CAD build for the part. Positions are in the model's coordinates, mm. Face numbers are marked on the shaded views. Give positions to 0.01 mm unless a question says otherwise; leave off trailing zeros. Loops run counter-clockwise (first coordinate to the right, second up) from the corner with the lowest first, then second, coordinate; pieces in that order, holes last. Notation, with made-up numbers: M 48.5,61 L 79.5,61 A28 ccw 79.5,87 Z; hole C 16.25,48 d11. An arc over 180 degrees is marked long. Answer as CSV lines item,"result".
```python
from build123d import *

# Parameters (mm, degrees)
EXTRUDE_1_DEPTH     = 2.5
FILLET_1_R          = 5
FILLET_2_R          = 5
FILLET_3_R          = 5
FILLET_4_R          = 5
SKETCH_2_R          = 3.5
SKETCH_2_R_2        = 1.54
SKETCH_2_R_3        = 5
CUT_EXTRUDE_2_DEPTH = 2.5
FILLET_5_R          = 3
FILLET_6_R          = 3
FILLET_7_R          = 3
FILLET_8_R          = 3
FILLET_9_R          = 3
FILLET_10_R         = 3
FILLET_11_R         = 3
FILLET_12_R         = 3


with BuildPart() as part:
    # 草图1 → 凸台-拉伸1 (new body)
    with BuildSketch(Plane.XY):
        Polygon((0, 13.5), (13.5, 0), (0, -13.5), (-13.5, 0), align=None)
    extrude(amount=EXTRUDE_1_DEPTH)

    # 圆角1
    fillet_1_edges = [part.edges().sort_by_distance(p)[0] for p in [
        (13.5, 0, 1.25),
    ]]
    fillet(fillet_1_edges, radius=FILLET_1_R)

    # 圆角2
    fillet_2_edges = [part.edges().sort_by_distance(p)[0] for p in [
        (0, -13.5, 1.25),
    ]]
    fillet(fillet_2_edges, radius=FILLET_2_R)

    # 圆角3
    fillet_3_edges = [part.edges().sort_by_distance(p)[0] for p in [
        (-13.5, 0, 1.25),
    ]]
    fillet(fillet_3_edges, radius=FILLET_3_R)

    # 圆角4
    fillet_4_edges = [part.edges().sort_by_distance(p)[0] for p in [
        (0, 13.5, 1.25),
    ]]
    fillet(fillet_4_edges, radius=FILLET_4_R)

    # 草图2 → 切除-拉伸2 (cut)
    with BuildSketch(Plane(origin=(0, 0, 0), x_dir=(-1, 0, 0), z_dir=(0, 0, -1))):
        Circle(SKETCH_2_R)
        with Locations((0, -6)):
            Circle(SKETCH_2_R_2)
        with Locations((0, 6)):
            Circle(SKETCH_2_R_2)
        with Locations((8, 0)):
            Circle(SKETCH_2_R_2)
        with Locations((-8, 0)):
            Circle(SKETCH_2_R_2)
        with Locations((8, 8)):
            Circle(SKETCH_2_R_3)
        with Locations((8, -8)):
            Circle(SKETCH_2_R_3)
        with Locations((-8, -8)):
            Circle(SKETCH_2_R_3)
        with Locations((-8, 8)):
            Circle(SKETCH_2_R_3)
    extrude(amount=-CUT_EXTRUDE_2_DEPTH, mode=Mode.SUBTRACT)

    # 圆角5
    fillet_5_edges = [part.edges().sort_by_distance(p)[0] for p in [
        (3.442062075, -10.055529584, 1.25),
    ]]
    fillet(fillet_5_edges, radius=FILLET_5_R)

    # 圆角6
    fillet_6_edges = [part.edges().sort_by_distance(p)[0] for p in [
        (-3.442062075, -10.055529584, 1.25),
    ]]
    fillet(fillet_6_edges, radius=FILLET_6_R)

    # 圆角7
    fillet_7_edges = [part.edges().sort_by_distance(p)[0] for p in [
        (-10.055529584, -3.442062075, 1.25),
    ]]
    fillet(fillet_7_edges, radius=FILLET_7_R)

    # 圆角8
    fillet_8_edges = [part.edges().sort_by_distance(p)[0] for p in [
        (3.442062075, 10.055529584, 1.25),
    ]]
    fillet(fillet_8_edges, radius=FILLET_8_R)

    # 圆角9
    fillet_9_edges = [part.edges().sort_by_distance(p)[0] for p in [
        (-3.442062075, 10.055529584, 1.25),
    ]]
    fillet(fillet_9_edges, radius=FILLET_9_R)

    # 圆角10
    fillet_10_edges = [part.edges().sort_by_distance(p)[0] for p in [
        (-10.055529584, 3.442062075, 1.25),
    ]]
    fillet(fillet_10_edges, radius=FILLET_10_R)

    # 圆角11
    fillet_11_edges = [part.edges().sort_by_distance(p)[0] for p in [
        (10.055529584, -3.442062075, 1.25),
    ]]
    fillet(fillet_11_edges, radius=FILLET_11_R)

    # 圆角12
    fillet_12_edges = [part.edges().sort_by_distance(p)[0] for p in [
        (10.055529584, 3.442062075, 1.25),
    ]]
    fillet(fillet_12_edges, radius=FILLET_12_R)


solid = part.part
```
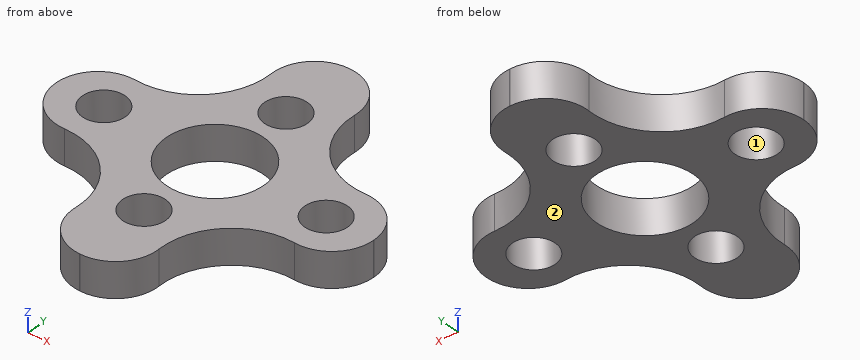
Q1. Cut at C-C (x = -0.5). Give the number of separate pieces and of enclosed holes in the cut face, and give its area (3 significant figures).
Solution:
separate pieces,"4"
enclosed holes,"0"
area,"25.1 mm²"
Q2. Pin check, flat tips, straight feed: P1, Ø1, axis at x = 5.5, z = 0.5, coming from the -Y side; P2, Ø1.8, axis at x = -8, y = 0, coming from the -Z side. Stop position of each tip, or through.
Solution:
P1,"stops at y = -4"
P2,"passes through"
Q3. Cut at A-A (x = 8). Write the cut outline in (y, z), and give its area (3 significant figures).
Solution:
outline,"M -3,0 L -1.54,0 L -1.54,2.5 L -3,2.5 Z; M 1.54,0 L 3,0 L 3,2.5 L 1.54,2.5 Z"
area,"7.30 mm²"
Q4. Cut at B-B (y = -6). Write the cut outline in (x, z).
Solution:
outline,"M -3.42,0 L -1.54,0 L -1.54,2.5 L -3.42,2.5 Z; M 1.54,0 L 3.42,0 L 3.42,2.5 L 1.54,2.5 Z"
Q5. Wall check: line 1 (Y direction, x = 0, z = 1.8); line 2 (X direction, y = -0.5, z = 1.5); line 3 (X direction, y = -1.25, z = 1.9). Give the ranges that are in metal, low to high. Write a range as [from, to].
Solution:
line 1,"y = [-11.43, -7.54], [-4.46, -3.5], [3.5, 4.46], [7.54, 11.43]"
line 2,"x = [-11.39, -9.46], [-6.54, -3.46], [3.46, 6.54], [9.46, 11.39]"
line 3,"x = [-11.16, -8.9], [-7.1, -3.27], [3.27, 7.1], [8.9, 11.16]"
Q6. Mould opens along X. For the marked faces 1 and 2 say: released by +X, released by -X, zero draft, split by the parting line, or undercut.
Solution:
face 1,"undercut"
face 2,"zero draft"
